```python
from build123d import *

# Parameters (mm, degrees)
SKETCH_1_W             = 41
SKETCH_1_H             = 41
SKETCH_1_W_2           = 25
SKETCH_1_H_2           = 35
EXTRUDE_1_DEPTH        = 72
SKETCH_2_W             = 41
SKETCH_2_H             = 41
EXTRUDE_2_DEPTH        = 3
CHAMFER_1_SIZE         = 3
FILLET_1_R             = 5
SKETCH_3_W             = 15
SKETCH_3_H             = 3
CUT_EXTRUDE_1_DEPTH    = 5
FILLET_2_R             = 3
SKETCH_4_W             = 3.5
SKETCH_4_H             = 28
CUT_EXTRUDE_2_DEPTH    = 6
SKETCH_6_W             = 3.5
SKETCH_6_H             = 3.5
CUT_EXTRUDE_4_DEPTH    = 83.428757118
SKETCH_7_W             = 3.5
SKETCH_7_H             = 3.5
CUT_EXTRUDE_5_DEPTH    = 83.428757118
FILLET_2_OF_MIRROR_1_R = 3
SKETCH_8_R             = 1.3
CUT_EXTRUDE_6_DEPTH    = 2.5


with BuildPart() as part:
    # ｽｹｯﾁ1 → ﾎﾞｽ - 押し出し1 (new body)
    with BuildSketch(Plane.XY):
        Rectangle(SKETCH_1_W, SKETCH_1_H)
        Rectangle(SKETCH_1_W_2, SKETCH_1_H_2, mode=Mode.SUBTRACT)
    extrude(amount=EXTRUDE_1_DEPTH)

    # ｽｹｯﾁ2 → ﾎﾞｽ - 押し出し2 (add)
    with BuildSketch(Plane(origin=(0, 0, 0), x_dir=(-1, 0, 0), z_dir=(0, 0, -1))):
        Rectangle(SKETCH_2_W, SKETCH_2_H)
    extrude(amount=EXTRUDE_2_DEPTH)

    # 面取り1
    chamfer_1_edges = [part.edges().sort_by_distance(p)[0] for p in [
        (20.5, 0, -3),
        (0, -20.5, -3),
        (-20.5, 0, -3),
        (0, 20.5, -3),
    ]]
    chamfer(chamfer_1_edges, length=CHAMFER_1_SIZE)

    # ﾌｨﾚｯﾄ1
    # the kernel refuses this fillet: 5 mm, written as the material it takes off along each edge
    with BuildSketch(Plane(origin=(-20.5, 20.5, 84.5), x_dir=(0, -1, 0), z_dir=(0, 0, -1)), Plane(origin=(20.5, 20.5, -12.5), x_dir=(0, -1, 0), z_dir=(0, 0, 1)), Plane(origin=(20.5, -20.5, -12.5), x_dir=(-1, 0, 0), z_dir=(0, 0, 1)), Plane(origin=(-20.5, -20.5, 84.5), x_dir=(1, 0, 0), z_dir=(0, 0, -1))) as fillet_1_piece_1:
        with BuildLine():
            CenterArc((FILLET_1_R, -FILLET_1_R), FILLET_1_R, 90, 90)
            Line((0, -FILLET_1_R), (0, 0))
            Line((0, 0), (FILLET_1_R, 0))
        make_face()
    extrude(amount=97, mode=Mode.SUBTRACT)
    with BuildSketch(Plane(origin=(-24.666666667, -24.666666667, 4.166666667), x_dir=(0.816496580927726, -0.40824829046386285, 0.4082482904638632), z_dir=(0.5773502691896258, 0.5773502691896258, -0.5773502691896258))) as fillet_1_piece_2:
        with BuildLine():
            CenterArc((FILLET_1_R * 0.57735026919, -FILLET_1_R), FILLET_1_R, 90, 60)
            Line((-FILLET_1_R * 0.288675134595, -FILLET_1_R * 0.5), (0, 0))
            Line((0, 0), (FILLET_1_R * 0.57735026919, 0))
        make_face()
    extrude(amount=19.629909152, mode=Mode.SUBTRACT)
    with BuildSketch(Plane(origin=(24.666666667, -24.666666667, 4.166666667), x_dir=(-0.816496580927726, -0.40824829046386285, 0.4082482904638632), z_dir=(-0.5773502691896258, 0.5773502691896258, -0.5773502691896258)), Plane(origin=(-13.333333333, 13.333333333, -7.166666667), x_dir=(-0.40824829046386285, -0.816496580927726, 0.4082482904638632), z_dir=(-0.5773502691896258, 0.5773502691896258, 0.5773502691896258)), Plane(origin=(24.666666667, 24.666666667, 4.166666667), x_dir=(0.40824829046386285, -0.816496580927726, 0.4082482904638632), z_dir=(-0.5773502691896258, -0.5773502691896258, -0.5773502691896258))) as fillet_1_piece_3:
        with BuildLine():
            CenterArc((FILLET_1_R * 0.57735026919, FILLET_1_R), FILLET_1_R, 210, 60)
            Line((-FILLET_1_R * 0.288675134595, FILLET_1_R * 0.5), (0, 0))
            Line((0, 0), (FILLET_1_R * 0.57735026919, 0))
        make_face()
    extrude(amount=19.629909152, mode=Mode.SUBTRACT)

    # ｽｹｯﾁ3 → ｶｯﾄ - 押し出し1 (cut)
    with BuildSketch(Plane.XY.offset(72)):
        with Locations((0, 19)):
            Rectangle(SKETCH_3_W, SKETCH_3_H)
    cut_extrude_1 = extrude(amount=-CUT_EXTRUDE_1_DEPTH, mode=Mode.SUBTRACT)

    # ﾌｨﾚｯﾄ2
    fillet_2_edges = [part.edges().sort_by_distance(p)[0] for p in [
        (-7.5, 19, 67),
        (7.5, 19, 67),
    ]]
    fillet(fillet_2_edges, radius=FILLET_2_R)

    # ｽｹｯﾁ4 → ｶｯﾄ - 押し出し2 (cut)
    with BuildSketch(Plane.XY.offset(72)):
        with Locations((-16.5, 0)):
            Rectangle(SKETCH_4_W, SKETCH_4_H)
        with Locations((16.5, 0)):
            Rectangle(SKETCH_4_W, SKETCH_4_H)
    extrude(amount=-CUT_EXTRUDE_2_DEPTH, mode=Mode.SUBTRACT)

    # ｽｹｯﾁ6 → ｶｯﾄ - 押し出し4 (cut, through all)
    with BuildSketch(Plane.XZ.offset(-14)):
        with Locations((16.5, 67.75)):
            Rectangle(SKETCH_6_W, SKETCH_6_H)
    extrude(amount=-CUT_EXTRUDE_4_DEPTH, mode=Mode.SUBTRACT)

    # ｽｹｯﾁ7 → ｶｯﾄ - 押し出し5 (cut, through all)
    with BuildSketch(Plane(origin=(0, -14, 0), x_dir=(1, 0, 0), z_dir=(0, 1, 0))):
        with Locations((-16.5, -67.75)):
            Rectangle(SKETCH_7_W, SKETCH_7_H)
    extrude(amount=-CUT_EXTRUDE_5_DEPTH, mode=Mode.SUBTRACT)

    # ﾐﾗｰ1: ｶｯﾄ - 押し出し1 across plane
    add(cut_extrude_1.mirror(Plane.ZX), mode=Mode.SUBTRACT)

    # ﾌｨﾚｯﾄ2 of ﾐﾗｰ1
    fillet_2_of_mirror_1_edges = [part.edges().sort_by_distance(p)[0] for p in [
        (-7.5, -19, 67),
        (7.5, -19, 67),
    ]]
    fillet(fillet_2_of_mirror_1_edges, radius=FILLET_2_OF_MIRROR_1_R)

    # ｽｹｯﾁ8 → ｶｯﾄ - 押し出し6 (cut)
    with BuildSketch(Plane.XY.offset(72)):
        with Locations((17, 17)):
            Circle(SKETCH_8_R)
        with Locations((17, -17)):
            Circle(SKETCH_8_R)
        with Locations((-17, -17)):
            Circle(SKETCH_8_R)
        with Locations((-17, 17)):
            Circle(SKETCH_8_R)
    extrude(amount=-CUT_EXTRUDE_6_DEPTH, mode=Mode.SUBTRACT)


solid = part.part
```
Here's how the part is built. I have some questions about the finished solid (model axes, mm). A direction names the side the tool comes from. Give positions to 0.01 mm unless a question says otherwise; leave off trailing zeros. Write each loop counter-clockwise with the first axis right and the second up, starting at its lowest first coordinate (ties: lowest second). Pieces come first, ordered by that corner, then holes. Notation, with made-up numbers: M 28.25,-19 L 65.25,-19 A22 ccw 65.25,10 Z; hole C 41.25,80.5 d10. An arc over 180 degrees is marked long. Put each result on its own line as item: value. Start each with the question number.
Item 1: I need wall thicknesses on L1, parallel to X at y = -6, z = 68; L2, parallel to Y at x = 6, z = 1; L3, parallel to X at y = 15, z = 31.5. Which ranges of each line are inside material? Lowest first, please. Write a range as from..to.
Item 2: On a 3-axis mill with a long thin cutter (end or side, diameter ignored), from which of +Z, -Z, +X, -X, +Y, -Y can I reach the whole of each face in a straight line? I mean faces 4 (the flat face through (-14, 0, 72)), 5 (the flat face through (-14.75, -3, 69)), 6 (the flat face through (16, 14, 71)), 7 (the cylindrical face through (-19.07, 19, 36.21)), 8 (the flat face through (-7.5, -19, 71)). Say none if no direction works.
Item 3: Thinking about a two-plate mould opening in Y: for faces 1 (the flat face through (0, -17.5, 35)), 2 (the flat face through (20.5, 0, 37)), 3 (the cylindrical face through (-17.5, -17.6, -2)), which applies, +Y half, -Y half, draft (parallel to the pull), parting line (faces both ways), or undercut?
Item 4: If we section it at B-B, the plane y = 8: Write out the boundary of the cut face in (x, z), then the cut area to 3 significant figures.
Item 5: If we section it at A-A, the plane z = 49.5: Write out the boundary of the cut face in (x, y).
Item 6: Will these pins go through, and if not, where does the flat tip stop? pin 1 (20 mm diameter, centred on x = 1.5, y = -6, fed in from +Z); pin 2 (1 mm diameter, centred on x = 17, y = 11, fed in from +Z); pin 3 (4 mm diameter, centred on x = -1, y = -16.5, fed in from +Z).
Item 7: If we section it at C-C, the plane x = 3.5: Write out the boundary of the cut face in (y, z).
Values:
1. L1: -20.5..-18.25, -14.75..-12.5, 12.5..14.75, 18.25..20.5
1. L2: -20.5..-17.5, 17.5..20.5
1. L3: -20.5..-12.5, 12.5..20.5
2. face 4: +Z, +X, -X, +Y, -Y
2. face 5: none
2. face 6: +Z
2. face 7: +Z, -Z, -X, +Y
2. face 8: +Z, +Y, -Y
3. face 1: undercut
3. face 2: draft
3. face 3: -Y half
4. outline: M -20.5,0 L -17.5,-3 L 17.5,-3 L 20.5,0 L 20.5,72 L 18.25,72 L 18.25,66 L 14.75,66 L 14.75,72 L 12.5,72 L 12.5,0 L -12.5,0 L -12.5,72 L -14.75,72 L -14.75,66 L -18.25,66 L -18.25,72 L -20.5,72 Z
4. area: 1,220 mm²
5. outline: M -20.5,-15.5 A5 ccw -15.5,-20.5 L 15.5,-20.5 A5 ccw 20.5,-15.5 L 20.5,15.5 A5 ccw 15.5,20.5 L -15.5,20.5 A5 ccw -20.5,15.5 Z; hole M -12.5,-17.5 L 12.5,-17.5 L 12.5,17.5 L -12.5,17.5 Z
6. pin 1: z = 0
6. pin 2: z = 66
6. pin 3: z = 67
7. outline: M -20.5,0 L -17.5,-3 L 17.5,-3 L 20.5,0 L 20.5,67 L 17.5,67 L 17.5,0 L -17.5,0 L -17.5,67 L -20.5,67 Z
